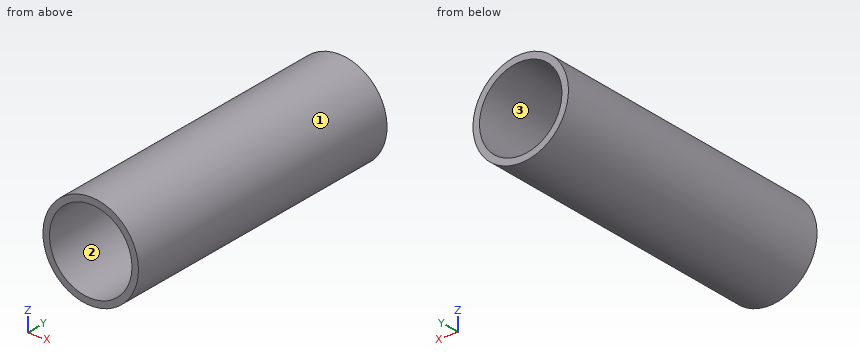
```python
from build123d import *

# Parameters (mm, degrees)
SKETCH3_R           = 11
BOSS_EXTRUDE1_DEPTH = 70
SKETCH4_R           = 2.8
CUT_EXTRUDE1_DEPTH  = 70
SKETCH5_R           = 9.5
CUT_EXTRUDE2_DEPTH  = 33.5
CUT_EXTRUDE3_START  = -33.5
SKETCH6_R           = 9.5
CUT_EXTRUDE3_DEPTH  = 33.5


with BuildPart() as part:
    # Sketch3 → Boss-Extrude1 (new body)
    with BuildSketch(Plane(origin=(0, 0, 0), x_dir=(1, 0, 0), z_dir=(0, 1, 0))):
        with Locations(Location((0, 0, 0), (0, 0, 270))):
            Circle(SKETCH3_R)
    extrude(amount=BOSS_EXTRUDE1_DEPTH)

    # Sketch4 → Cut-Extrude1 (cut)
    with BuildSketch(Plane(origin=(0, 70, 0), x_dir=(1, 0, 0), z_dir=(0, 1, 0))):
        with Locations(Location((0, 0, 0), (0, 0, 270))):
            Circle(SKETCH4_R)
    extrude(amount=-CUT_EXTRUDE1_DEPTH, mode=Mode.SUBTRACT)

    # Sketch5 → Cut-Extrude2 (cut)
    with BuildSketch(Plane(origin=(0, 0, 0), x_dir=(-1, 0, 0), z_dir=(0, -1, 0))):
        with Locations(Location((0, 0, 0), (0, 0, 90))):
            Circle(SKETCH5_R)
    extrude(amount=-CUT_EXTRUDE2_DEPTH, mode=Mode.SUBTRACT)

    # Sketch6 → Cut-Extrude3 (cut)
    with BuildSketch(Plane(origin=(0, 70, 0), x_dir=(1, 0, 0), z_dir=(0, 1, 0)).offset(CUT_EXTRUDE3_START)):
        with Locations(Location((0, 0, 0), (0, 0, 90))):
            Circle(SKETCH6_R)
    extrude(amount=CUT_EXTRUDE3_DEPTH, mode=Mode.SUBTRACT)


solid = part.part
```
The model under review builds one solid part; all positions refer to its coordinate system, in mm. Face numbers are marked on the shaded views. Coordinates: 2 decimals unless noted, no trailing zeros. Write each loop counter-clockwise with the first axis right and the second up, starting at its lowest first coordinate (ties: lowest second). Pieces come first, ordered by that corner, then holes.
1) We need section D-D on x = 4.75. State the section outline as (y, z) points.
2) We need section A-A on x = 0. State the section outline as (y, z) points.
3) We need section B-B on z = 0. State the section outline as (x, y) points.
4) Clearance check with flat-ended pins moving along their axes: pin 1 Ø4 at (x, z) = (-4.5, 3) entering from -Y; pin 2 Ø1.5 at (x, z) = (-0.5, 4) entering from +Y; pin 3 Ø8 at (x, y) = (8, 40.5) entering from +Z; pin 4 Ø3.5 at (x, z) = (0, 0) entering from -Y. State where each tip first meets the part, or that it passes through.
5) The part is to be moulded in two halves that separate along X. For the marked faces 1, 2 and 3, say which applies: pulls with the +X half, pulls with the -X half, needs draft (parallel to the pull), parting line crosses it, or undercut.
6) We need section C-C on y = 31. State the section outline as (x, z) points, then the cut area to 3 significant figures.
7) To check wall thickness, follow probe 1 along X at (y, z) = (34.2, 0); probe 2 along X at (y, z) = (60.5, 0); probe 3 along Y at (x, z) = (5.5, 4). State the ranges of each line that lie inside material, in increasing order.
Answer list:
1. outline: (0, -9.92) - (70, -9.92) - (70, -8.23) - (36.5, -8.23) - (36.5, 8.23) - (70, 8.23) - (70, 9.92) - (0, 9.92) - (0, 8.23) - (33.5, 8.23) - (33.5, -8.23) - (0, -8.23) - close
2. outline: (0, -11) - (70, -11) - (70, -9.5) - (36.5, -9.5) - (36.5, -2.8) - (33.5, -2.8) - (33.5, -9.5) - (0, -9.5) - close; (0, 9.5) - (33.5, 9.5) - (33.5, 2.8) - (36.5, 2.8) - (36.5, 9.5) - (70, 9.5) - (70, 11) - (0, 11) - close
3. outline: (-11, 0) - (-9.5, 0) - (-9.5, 33.5) - (-2.8, 33.5) - (-2.8, 36.5) - (-9.5, 36.5) - (-9.5, 70) - (-11, 70) - close; (2.8, 33.5) - (9.5, 33.5) - (9.5, 0) - (11, 0) - (11, 70) - (9.5, 70) - (9.5, 36.5) - (2.8, 36.5) - close
4. pin 1: stops at y = 33.5
4. pin 2: stops at y = 36.5
4. pin 3: stops at z = 10.25
4. pin 4: passes through
5. face 1: parting line crosses it
5. face 2: undercut
5. face 3: undercut
6. outline: circle Ø22 at (0, 0); hole circle Ø19 at (0, 0)
6. area: 96.6 mm2
7. probe 1: x = -11 to -2.8, 2.8 to 11
7. probe 2: x = -11 to -9.5, 9.5 to 11
7. probe 3: y = 33.5 to 36.5
